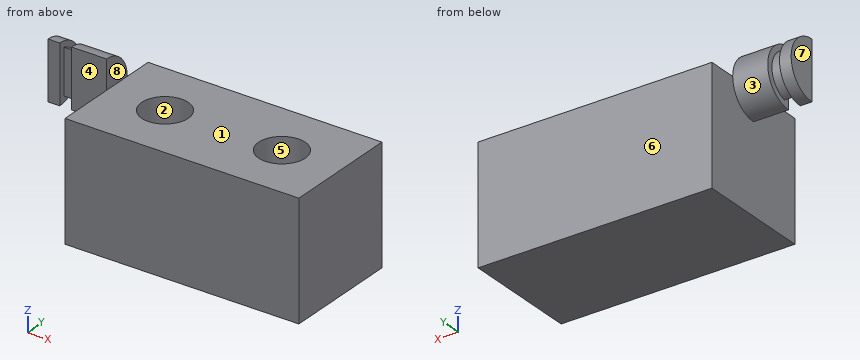
```python
from build123d import *

# Parameters (mm, degrees)
SKETCH1_W           = 50.8
SKETCH1_H           = 25.4
BOSS_EXTRUDE1_DEPTH = 25.4
SKETCH2_R           = 5.08
CUT_EXTRUDE1_DEPTH  = 13.97
BOSS_EXTRUDE2_DEPTH = 12.7
CUT_EXTRUDE3_START  = -7.62
CUT_EXTRUDE3_DEPTH  = 2.54


with BuildPart() as part:
    # Sketch1 → Boss-Extrude1 (new body)
    with BuildSketch(Plane(origin=(0, 0, 0), x_dir=(1, 0, 0), z_dir=(0, 1, 0))):
        with Locations((25.4, 12.7)):
            Rectangle(SKETCH1_W, SKETCH1_H)
    extrude(amount=-BOSS_EXTRUDE1_DEPTH)

    # Sketch2 → Cut-Extrude1 (cut)
    with BuildSketch(Plane.XY):
        with Locations((12.7, -12.7)):
            Circle(SKETCH2_R)
        with Locations((38.1, -12.7)):
            Circle(SKETCH2_R)
    extrude(amount=-CUT_EXTRUDE1_DEPTH, mode=Mode.SUBTRACT)

    # Sketch3 → Boss-Extrude2 (add)
    with BuildSketch(Plane(origin=(0, 0, 0), x_dir=(0, 0, -1), z_dir=(1, 0, 0))):
        with BuildLine():
            Line((-6.35, -12.7), (6.35, -12.7))
            ThreePointArc((6.35, -12.7), (0, -6.35), (-6.35, -12.7))
        make_face()
    extrude(amount=-BOSS_EXTRUDE2_DEPTH)

    # Sketch4 → Cut-Extrude3 (cut)
    with BuildSketch(Plane(origin=(0, 0, 0), x_dir=(0, 0, -1), z_dir=(1, 0, 0)).offset(CUT_EXTRUDE3_START)):
        with BuildLine():
            Line((-6.35, -12.7), (6.35, -12.7))
            ThreePointArc((6.35, -12.7), (0, -6.35), (-6.35, -12.7))
        make_face()
        with BuildLine():
            Line((-4.91868885, -11.43), (4.91868885, -11.43))
            ThreePointArc((4.91868885, -11.43), (0, -7.62), (-4.91868885, -11.43))
        make_face(mode=Mode.SUBTRACT)
    extrude(amount=-CUT_EXTRUDE3_DEPTH, mode=Mode.SUBTRACT)


solid = part.part
```
Build history of the part. All positions in model axes, mm. Face numbers are marked on the shaded views. A direction names the side the tool comes from. Round coordinates to 2 decimals unless told otherwise and drop trailing zeros. Loops run counter-clockwise (first coordinate to the right, second up) from the corner with the lowest first, then second, coordinate; pieces in that order, holes last.
Item 1: Which spindle directions (+Z, -Z, +X, -X, +Y, -Y) get a long thin tool onto all of the face, cutting with end or side? Do the marked faces 1, 2, 3 and 4. Say none if no direction does.
Item 2: Drill centre lines: line 1 along Y through (x, z) = (38.1, -6.75); line 2 along X through (y, z) = (-10.25, -4); line 3 along X through (y, z) = (-10.75, -22). Where is each one in solid material? Low to high.
Item 3: Saw through at B-B (z = -4). List the corners of the cut face in (x, y).
Item 4: Saw through at A-A (x = 12.7). List the corners of the cut face in (y, z).
Item 5: Pin check, flat tips, straight feed: P1, Ø2, axis at x = -11, z = 2.5, coming from the -Y side; P2, Ø8, axis at x = 12.7, y = -12.7, coming from the +Z side; P3, Ø1.3, axis at x = -8.5, z = -2.5, coming from the -Y side; P4, Ø2, axis at x = -2, z = -17, coming from the -Y side. Stop position of each tip, or through.
Item 6: Saw through at C-C (y = -9.5). List the corners of the cut face in (x, z).
Item 7: Saw through at D-D (z = -21). List the corners of the cut face in (x, y), then the cut area to 3 significant figures.
Item 8: Two-plate mould, pull along X, no slides. Class the marked faces 5, 6, 7 and 8: released by +X, released by -X, zero draft, split by the parting line, or undercut.
Worked answers:
1. face 1: +Z, +X, +Y, -Y
1. face 2: +Z
1. face 3: -X, +Y
1. face 4: +Z, -Z, -X, -Y
2. line 1: y = -25.4 to -17.78, -7.62 to 0
2. line 2: x = -12.7 to 8.25, 17.15 to 33.65, 42.55 to 50.8
2. line 3: x = 0 to 50.8
3. outline: (-12.7, -12.7) - (-10.16, -12.7) - (-10.16, -11.43) - (-7.62, -11.43) - (-7.62, -12.7) - (0, -12.7) - (0, -25.4) - (50.8, -25.4) - (50.8, 0) - (0, 0) - (0, -7.77) - (-7.62, -7.77) - (-7.62, -9.57) - (-10.16, -9.57) - (-10.16, -7.77) - (-12.7, -7.77) - close; hole circle Ø10.16 at (12.7, -12.7); hole circle Ø10.16 at (38.1, -12.7)
4. outline: (-25.4, -25.4) - (0, -25.4) - (0, 0) - (-7.62, 0) - (-7.62, -13.97) - (-17.78, -13.97) - (-17.78, 0) - (-25.4, 0) - close
5. P1: stops at y = -12.7
5. P2: stops at z = -13.97
5. P3: stops at y = -11.43
5. P4: passes through
6. outline: (-12.7, -5.48) - (-10.16, -5.48) - (-10.16, -3.95) - (-7.62, -3.95) - (-7.62, -5.48) - (0, -5.48) - (0, -25.4) - (50.8, -25.4) - (50.8, 0) - (42.05, 0) - (42.05, -13.97) - (34.15, -13.97) - (34.15, 0) - (16.65, 0) - (16.65, -13.97) - (8.75, -13.97) - (8.75, 0) - (0, 0) - (0, 5.48) - (-7.62, 5.48) - (-7.62, 3.95) - (-10.16, 3.95) - (-10.16, 5.48) - (-12.7, 5.48) - close
7. outline: (0, -25.4) - (50.8, -25.4) - (50.8, 0) - (0, 0) - close
7. area: 1,290 mm2
8. face 5: undercut
8. face 6: zero draft
8. face 7: released by -X
8. face 8: released by +X
